Check sheet for the modelled part. Datum: model origin and axes. Units: mm. A direction names the side the tool comes from. Give positions to 0.01 mm unless a question says otherwise; leave off trailing zeros. Write each loop counter-clockwise with the first axis right and the second up, starting at its lowest first coordinate (ties: lowest second). Pieces come first, ordered by that corner, then holes.
from build123d import *

# Parameters (mm, degrees)
BOSS_EXTRUDE1_DEPTH = 4
BOSS_EXTRUDE1_DRAFT = -2
SHELL1_T            = -0.5


with BuildPart() as part:
    # Sketch1 → Boss-Extrude1 (with draft: the straight prism first)
    with BuildSketch(Plane(origin=(0, 0, 0), x_dir=(1, 0, 0), z_dir=(0, 1, 0))):
        with BuildLine():
            Line((-7.5, -6.375), (7.5, -6.375))
            ThreePointArc((7.5, -6.375), (8.207106781, -6.082106781), (8.5, -5.375))
            Line((8.5, -5.375), (8.5, 5.375))
            ThreePointArc((8.5, 5.375), (8.207106781, 6.082106781), (7.5, 6.375))
            Line((7.5, 6.375), (-7.5, 6.375))
            ThreePointArc((-7.5, 6.375), (-8.207106781, 6.082106781), (-8.5, 5.375))
            Line((-8.5, 5.375), (-8.5, -5.375))
            ThreePointArc((-8.5, -5.375), (-8.207106781, -6.082106781), (-7.5, -6.375))
        make_face()
    extrude(amount=-BOSS_EXTRUDE1_DEPTH)
    # Boss-Extrude1: the draft: its side faces are tilted about the plane it starts from
    boss_extrude1_sides = [part.faces().sort_by_distance(p)[0] for p in [
        (0, -2, 6.375),
        (8.207106781, -2, 6.082106781),
        (8.5, -2, 0),
        (8.207106781, -2, -6.082106781),
        (0, -2, -6.375),
        (-8.207106781, -2, -6.082106781),
        (-8.5, -2, 0),
        (-8.207106781, -2, 6.082106781),
    ]]
    draft(boss_extrude1_sides, Plane(origin=(0, 0, 0), x_dir=(1, 0, 0), z_dir=(0, 1, 0)), BOSS_EXTRUDE1_DRAFT)

    # Shell1
    shell1_openings = [part.faces().sort_by_distance(p)[0] for p in [
        (0, 0, 0),
    ]]
    offset(amount=SHELL1_T, openings=shell1_openings, kind=Kind.INTERSECTION)


solid = part.part
1) Access from +Z, -Z, +X, -X, +Y, -Y to the whole of each face (thin tool, end or side, straight path). Record for faces 4 (the conical face through (8.166, -1.972, -6.026)), 5 (the conical face through (-8.166, -1.972, 6.026)).
2) Sectioned sample at A-A on x = -7.25. Record the boundary of the cut face in (y, z) (3 decimals).
3) Sectioned sample at B-B on z = -5. Record the boundary of the cut face in (x, y), then the cut area to 3 significant figures.
4) Sectioned sample at D-D on y = -2.25. Record the boundary of the cut face in (x, z) (3 decimals).
5) Gauge pin test, flat ends, axial feed: pin 1 (6 mm diameter, centred on x = -4, z = -1, fed in from +Y); pin 2 (1.5 mm diameter, centred on x = -5.5, y = -1.5, fed in from -Z). Record the tip position at first contact, or that the pin passes through.
6) Sectioned sample at C-C on y = -0.8. Record the boundary of the cut face in (x, z) (3 decimals).
7) Scan lines: L1, parallel to Y at x = -1.25, z = 1; L2, parallel to X at y = -1.55, z = -5; L3, parallel to Z at x = -4, y = -3.4. Record each from-to range of solid material in increasing order.
8) Draft check along X on faces 1 (the flat face through (0, 0, 6.1)), 2 (the conical face through (8.15, -1.97, 6.04)), 3 (the flat face through (0, -3.5, 0)). Enter one of: +X half, -X half, draft (parallel to the pull), parting line (faces both ways), or undercut.
Answers below:
1. face 4: -Z, +X, -Y
1. face 5: +Z, -X, -Y
2. outline: (-4, -6.235) - (0, -6.375) - (0, -5.875) - (-3.5, -5.752) - (-3.5, 5.752) - (0, 5.875) - (0, 6.375) - (-4, 6.235) - close
3. outline: (-8.5, 0) - (-8.36, -4) - (8.36, -4) - (8.5, 0) - (8, 0) - (7.88, -3.5) - (-7.88, -3.5) - (-8, 0) - close
3. area: 11.9 mm2
4. outline: (-8.421, -5.375) arc R0.921 ccw to (-7.5, -6.296) - (7.5, -6.296) arc R0.921 ccw to (8.421, -5.375) - (8.421, 5.375) arc R0.921 ccw to (7.5, 6.296) - (-7.5, 6.296) arc R0.921 ccw to (-8.421, 5.375) - close; hole (-7.921, -5.375) arc R0.421 ccw to (-7.5, -5.796) - (7.5, -5.796) arc R0.421 ccw to (7.921, -5.375) - (7.921, 5.375) arc R0.421 ccw to (7.5, 5.796) - (-7.5, 5.796) arc R0.421 ccw to (-7.921, 5.375) - close
5. pin 1: stops at y = -3.5
5. pin 2: stops at z = -6.35
6. outline: (-8.472, -5.375) arc R0.972 ccw to (-7.5, -6.347) - (7.5, -6.347) arc R0.972 ccw to (8.472, -5.375) - (8.472, 5.375) arc R0.972 ccw to (7.5, 6.347) - (-7.5, 6.347) arc R0.972 ccw to (-8.472, 5.375) - close; hole (-7.972, -5.375) arc R0.472 ccw to (-7.5, -5.847) - (7.5, -5.847) arc R0.472 ccw to (7.972, -5.375) - (7.972, 5.375) arc R0.472 ccw to (7.5, 5.847) - (-7.5, 5.847) arc R0.472 ccw to (-7.972, 5.375) - close
7. L1: y = -4 to -3.5
7. L2: x = -8.45 to -7.95, 7.95 to 8.45
7. L3: z = -6.26 to -5.76, 5.76 to 6.26
8. face 1: draft
8. face 2: +X half
8. face 3: undercut
